from build123d import *

# Parameters (mm, degrees)
F_4_40_TAPPED_HOLE1_D           = 2.2606
F_4_40_TAPPED_HOLE1_DEPTH       = 8.763
F_4_40_TAPPED_HOLE1_CSINK_D     = 3.302
F_4_40_TAPPED_HOLE1_CSINK_ANGLE = 82
F_4_40_TAPPED_HOLE1_TIP         = 0.679152758
F_3_32_0_09375_DIAMETER_HOLE1_D = 2.38125
CUT_EXTRUDE1_DEPTH              = 26.043807596
CIRPATTERN1_COUNT               = 2
CHAMFER1_SIZE                   = 1.016
CHAMFER1_SIZE2                  = 1.75976362


with BuildPart() as part:
    # Sketch1 → Revolve1 (revolve)
    with BuildSketch(Plane.XY, mode=Mode.PRIVATE) as revolve1_sk:
        Polygon((0, 0), (3.175, 0), (3.175, 2.54), (2.54, 2.54), (2.54, 24.638), (0, 24.638), align=None)
    revolve(revolve1_sk.sketch.rotate(Axis((0, 0, 0), (0, 1, 0)), 90), axis=Axis((0, 0, 0), (0, 1, 0)))

    # 4-40 Tapped Hole1
    with Locations(Plane.XZ):
        with Locations((0, 0)):
            CounterSinkHole(F_4_40_TAPPED_HOLE1_D / 2, F_4_40_TAPPED_HOLE1_CSINK_D / 2, depth=F_4_40_TAPPED_HOLE1_DEPTH, counter_sink_angle=F_4_40_TAPPED_HOLE1_CSINK_ANGLE)
            with Locations((0, 0, -(F_4_40_TAPPED_HOLE1_DEPTH + F_4_40_TAPPED_HOLE1_TIP / 2))):  # 118° drill point
                Cone(0, F_4_40_TAPPED_HOLE1_D / 2, F_4_40_TAPPED_HOLE1_TIP, mode=Mode.SUBTRACT)

    # 3_32 _0.09375_ Diameter Hole1 (through all)
    with Locations(Plane.XY.offset(2.54)):
        with Locations((0, 8.128)):
            Hole(F_3_32_0_09375_DIAMETER_HOLE1_D / 2)

    # Sketch6 → Cut-Extrude1 (cut, symmetric)
    with BuildSketch(Plane(origin=(0, 0, 0), x_dir=(0, 0, -1), z_dir=(1, 0, 0))):
        with BuildLine():
            Line((1.27, 24.638), (1.27, 12.7))
            ThreePointArc((1.27, 12.7), (1.605193669, 11.280096834), (2.54, 10.16))
            Line((2.54, 10.16), (2.54, 24.638))
            Line((2.54, 24.638), (1.27, 24.638))
        make_face()
    cut_extrude1 = extrude(amount=CUT_EXTRUDE1_DEPTH, both=True, mode=Mode.SUBTRACT)

    # CirPattern1: Cut-Extrude1 ×2 about axis
    cirpattern1_axis = Axis((0, -1.2319, 0), (0, 1, 0))
    for i in range(1, CIRPATTERN1_COUNT):
        add(cut_extrude1.rotate(cirpattern1_axis, i * 360 / CIRPATTERN1_COUNT), mode=Mode.SUBTRACT)

    # Chamfer1
    chamfer1_edges = [part.edges().sort_by_distance(p)[0] for p in [
        (0, 24.638, -1.27),
        (0, 24.638, 1.27),
    ]]
    chamfer1_side = [part.faces().sort_by_distance(p)[0] for p in [
        (0, 24.638, 0),
    ]]
    chamfer(chamfer1_edges, length=CHAMFER1_SIZE, length2=CHAMFER1_SIZE2, reference=chamfer1_side[0])


solid = part.part
Can you work these out from the model? Positions are in its coordinate system, mm. A direction names the side the tool comes from. Coordinates: 2 decimals unless noted, no trailing zeros. Loops run counter-clockwise (first coordinate to the right, second up) from the corner with the lowest first, then second, coordinate; pieces in that order, holes last. Notation, with made-up numbers: (42, 59) - (66, 59) arc R22 cw to (66, 71) - close; hole circle Ø10 at (8.5, 69). An arc over 180 degrees is marked (long way). Answer as a JSON object with one key per item and string values. Group by question number.
Item 1: On a 3-axis mill with a long thin cutter (end or side, diameter ignored), from which of +Z, -Z, +X, -X, +Y, -Y can I reach the whole of each face in a straight line? I mean faces 1 (the face through (-3, 2.54, 0)), 2 (the face through (0, 18, -1.27)), 3 (the face through (0, 18, 1.27)). Say none if no direction works.
Item 2: For pin 1 (2 mm diameter, centred on x = -1, y = 19.5, fed in from -Z); pin 2 (2 mm diameter, centred on y = 5.5, z = -0.5, fed in from -X); pin 3 (2 mm diameter, centred on x = 0, y = 15.5, fed in from +Z), each with a flat end and sliding along its axis, tell me the tip position at first contact or that it passes through.
Item 3: If we section it at C-C (z = 2.75): List the corners of the cut face in (x, y) for me.
Item 4: If I drill on L1, parallel to X at y = 3, z = 0; L2, parallel to Z at x = 1.25, y = 16; L3, parallel to X at y = 16.75, z = -0.25, over which ranges is the centre line in solid material (lowest first)? Write a range as from..to.
Item 5: If we mould it in two halves opening along X, with no side actions, what happens to faces 4 (the face through (1.93, 1.29, 2.52)), 5 (the face through (0.035, 23.746, -0.769)), 6 (the face through (-1.044, 4.227, -0.433))? For each: released by +X, released by -X, zero draft, split by the parting line, or undercut.
Item 6: If we section it at A-A (y = 5): List the corners of the cut face in (x, z) for me.
Item 7: If we section it at B-B (y = 16.5): List the corners of the cut face in (x, z) for me, plus the area to 3 significant figures.
Returned:
{
 "1": {"face 1": "+Y", "face 2": "-Z, +X, -X, +Y", "face 3": "+Z, +X, -X, +Y"},
 "2": {"pin 1": "stops at z = -1.27", "pin 2": "stops at x = -2.54", "pin 3": "stops at z = 1.27"},
 "3": {"outline": "(-1.59, 0) - (1.59, 0) - (1.59, 2.54) - (-1.59, 2.54) - close"},
 "4": {"L1": "x = -2.54..-1.13, 1.13..2.54", "L2": "z = -1.27..1.27", "L3": "x = -2.53..2.53"},
 "5": {"face 4": "split by the parting line", "face 5": "zero draft", "face 6": "undercut"},
 "6": {"outline": "circle Ø5.08 at (0, 0); hole circle Ø2.26 at (0, 0)"},
 "7": {"outline": "(-2.2, -1.27) - (2.2, -1.27) arc R2.54 ccw to (2.2, 1.27) - (-2.2, 1.27) arc R2.54 ccw to start", "area": "12.3 mm²"}
}
